```python
from build123d import *

# Parameters (mm, degrees)
EXTRUDE_DEPTH = 188
FILLET_R      = 1
FILLET001_R   = 2
FILLET002_R   = 1


with BuildPart() as part:
    # Sketch → Extrude (new body)
    with BuildSketch(Plane.XY):
        Polygon((0, 0), (0, 60), (8.816349, 10), (106, 10), (106, 0), (86, 0), (86, -5), (71, -5), (71, 0), align=None)
    extrude(amount=EXTRUDE_DEPTH)

    # Fillet
    fillet_edges = [part.edges().sort_by_distance(p)[0] for p in [
        (4.408175, 35, 0),
        (4.408175, 35, 188),
    ]]
    fillet(fillet_edges, radius=FILLET_R)

    # Fillet001
    fillet001_edges = [part.edges().sort_by_distance(p)[0] for p in [
        (71, -5, 94),
        (86, -5, 94),
    ]]
    fillet(fillet001_edges, radius=FILLET001_R)

    # Fillet002
    fillet002_edges = [part.edges().sort_by_distance(p)[0] for p in [
        (71, -1.5, 0),
        (78.5, -5, 0),
        (86, -1.5, 0),
        (96, 0, 0),
        (106, 5, 0),
        (57.408175, 10, 0),
        (35.5, 0, 0),
        (71, -1.5, 188),
        (35.5, 0, 188),
        (0, 0, 94),
        (78.5, -5, 188),
        (86, -1.5, 188),
        (57.408175, 10, 188),
        (106, 10, 94),
        (106, 0, 94),
        (96, 0, 188),
        (106, 5, 188),
    ]]
    fillet(fillet002_edges, radius=FILLET002_R)


solid = part.part
```
Design review of the part built by this model. Coordinates are the model's own, in mm. A direction names the side the tool comes from. Round coordinates to 2 decimals unless told otherwise and drop trailing zeros. Order: outer loops, then holes, each group sorted by start corner. A loop starts at its lowest first (then second) coordinate and runs counter-clockwise, first axis right, second up. Notation, with made-up numbers: (-21, 7.5) - (-5, 7.5) arc R16 cw to (-5, 18.5) - close; hole circle Ø1 at (9, -36). An arc over 180 degrees is marked (long way). Return JSON: item names as keys, results as strings.
Q1. Machinability: for faces 1 (the flat face through (96, 0, 93)), 2 (the flat face through (36, 0, 93)), 3 (the flat face through (56, 10, 93)), which of the approach directions +Z, -Z, +X, -X, +Y, -Y give a long, thin tool a straight path to every point of the face, cutting with its end or side? Answer none if there is none.
Computed values:
{"face 1": "+Z, -Z, +X, -Y", "face 2": "+Z, -Z, -X, -Y", "face 3": "+Z, -Z, +X, +Y"}
Q2. Wall thickness on L1, parallel to Y at x = 101, z = 10; L2, parallel to Y at x = 76.5, z = 165; L3, parallel to X at y = 50.5, z = 20.5: over which ranges is each line inside the solid? List them lowest first. Write a range as [from, to].
Computed values:
{"L1": "y = [0, 10]", "L2": "y = [-5, 10]", "L3": "x = [0, 1.68]"}
Q3. Consider section B-B on x = 75.5. Write out the cut boundary in (y, z).
Computed values:
{"outline": "(-5, 1) arc R1 ccw to (-4, 0) - (9, 0) arc R1 ccw to (10, 1) - (10, 187) arc R1 ccw to (9, 188) - (-4, 188) arc R1 ccw to (-5, 187) - close"}
Q4. Consider section C-C on x = 31. Write out the cut boundary in (y, z), plus the area to 3 significant figures.
Computed values:
{"outline": "(0, 1) arc R1 ccw to (1, 0) - (9, 0) arc R1 ccw to (10, 1) - (10, 187) arc R1 ccw to (9, 188) - (1, 188) arc R1 ccw to (0, 187) - close", "area": "1,880 mm2"}
Q5. For pin 1 Ø0.9 at (y, z) = (-1.5, 122.5) entering from +X; pin 2 Ø12 at (y, z) = (29, 148.5) entering from +X; pin 3 Ø1 at (x, z) = (24, 145) entering from +Y, all flat-tipped, find the tip position at first contact; note any pin that passes through.
Computed values:
{"pin 1": "stops at x = 86", "pin 2": "stops at x = 6.52", "pin 3": "stops at y = 10"}
Q6. Consider section A-A on z = 29.5. Write out the cut boundary in (x, y), plus the area to 3 significant figures.
Computed values:
{"outline": "(0, 1) arc R1 ccw to (1, 0) - (71, 0) - (71, -3) arc R2 ccw to (73, -5) - (84, -5) arc R2 ccw to (86, -3) - (86, 0) - (105, 0) arc R1 ccw to (106, 1) - (106, 9) arc R1 ccw to (105, 10) - (8.82, 10) - (0, 60) - close", "area": "1,350 mm2"}
